```python
from build123d import *

# Parameters (mm, degrees)
DODANIE_WYCI_GNI_CIE2_DEPTH      = 3
DODANIE_WYCI_GNI_CIE2_DEPTH_BACK = 3
SZKIC2_W                         = 50
SZKIC2_H                         = 6
WYTNIJ_WYCI_GNI_CIE1_DEPTH       = 6
WYTNIJ_WYCI_GNI_CIE2_DEPTH       = 6
SZKIC4_W                         = 10
SZKIC4_H                         = 35
SZKIC4_H_2                       = 5
WYTNIJ_WYCI_GNI_CIE3_DEPTH       = 6
WYTNIJ_WYCI_GNI_CIE4_DEPTH       = 6
DODANIE_WYCI_GNI_CIE3_DEPTH      = 6
SZKIC8_R                         = 1.55
SZKIC8_R_2                       = 2.7
WYTNIJ_WYCI_GNI_CIE5_DEPTH       = 6


with BuildPart() as part:
    # Szkic1 → Dodanie-wyciągnięcie2 (new, two sides: drawn at the far end of the back side and taken through both)
    with BuildSketch(Plane(origin=(0, -418.87633849, -418.87633849), x_dir=(1, 0, 0), z_dir=(0, 1, 0)).offset(-DODANIE_WYCI_GNI_CIE2_DEPTH_BACK)):
        Polygon((-1165.368459045, -408.87633849), (-1142.368459045, -408.87633849), (-1142.368459045, -459.87633849), (-1100.368459045, -459.87633849), (-1100.368459045, -479.87633849), (-1165.368459045, -479.87633849), align=None)
    extrude(amount=DODANIE_WYCI_GNI_CIE2_DEPTH + DODANIE_WYCI_GNI_CIE2_DEPTH_BACK)

    # Szkic2 → Wytnij-wyciągnięcie1 (cut)
    with BuildSketch(Plane.XY.offset(61)):
        with Locations((-1140.368459045, -418.87633849)):
            Rectangle(SZKIC2_W, SZKIC2_H)
    extrude(amount=-WYTNIJ_WYCI_GNI_CIE1_DEPTH, mode=Mode.SUBTRACT)

    # Szkic3 → Wytnij-wyciągnięcie2 (cut)
    with BuildSketch(Plane(origin=(0, -415.87633849, 0), x_dir=(1, 0, 0), z_dir=(0, 1, 0))):
        Polygon((-1138.818459045, -55), (-1141.918459045, -55), (-1141.918459045, -51), (-1143.293459045, -51), (-1143.293459045, -49), (-1141.918459045, -49), (-1141.918459045, -48.5), (-1138.818459045, -48.5), (-1138.818459045, -49), (-1137.443459045, -49), (-1137.443459045, -51), (-1138.818459045, -51), align=None)
    extrude(amount=-WYTNIJ_WYCI_GNI_CIE2_DEPTH, mode=Mode.SUBTRACT)

    # Szkic4 → Wytnij-wyciągnięcie3 (cut)
    with BuildSketch(Plane(origin=(0, -415.87633849, 0), x_dir=(1, 0, 0), z_dir=(0, 1, 0))):
        with Locations((-1160.368459045, -17.5)):
            Rectangle(SZKIC4_W, SZKIC4_H)
        with Locations((-1160.368459045, -52.5)):
            Rectangle(SZKIC4_W, SZKIC4_H_2)
    extrude(amount=-WYTNIJ_WYCI_GNI_CIE3_DEPTH, mode=Mode.SUBTRACT)

    # Szkic5 → Wytnij-wyciągnięcie4 (cut)
    with BuildSketch(Plane(origin=(0, -415.87633849, 0), x_dir=(1, 0, 0), z_dir=(0, 1, 0))):
        Polygon((-1155.368459045, -8.168218351), (-1147.368459045, -8.168218351), (-1147.368459045, -6.793218351), (-1145.368459045, -6.793218351), (-1145.368459045, -8.168218351), (-1144.868459045, -8.168218351), (-1144.868459045, -11.268218351), (-1145.368459045, -11.268218351), (-1145.368459045, -12.643218351), (-1147.368459045, -12.643218351), (-1147.368459045, -11.268218351), (-1155.368459045, -11.268218351), align=None)
    extrude(amount=-WYTNIJ_WYCI_GNI_CIE4_DEPTH, mode=Mode.SUBTRACT)


with BuildPart() as body_2:
    # Szkic9 → Dodanie-wyciągnięcie3 (new body)
    with BuildSketch(Plane(origin=(0, -415.87633849, 0), x_dir=(1, 0, 0), z_dir=(0, 1, 0))):
        with BuildLine():
            Line((-1142.368459045, 10), (-1142.368459045, -41))
            Line((-1142.368459045, -41), (-1100.368459045, -41))
            Line((-1100.368459045, -41), (-1100.368459045, 0))
            ThreePointArc((-1100.368459045, 0), (-1103.297391233, 7.071067812), (-1110.368459045, 10))
            Line((-1110.368459045, 10), (-1142.368459045, 10))
        make_face()
    extrude(amount=-DODANIE_WYCI_GNI_CIE3_DEPTH)

    # Połącz3: union part
    add(part.part)

    # Szkic8 → Wytnij-wyciągnięcie5 (cut)
    with BuildSketch(Plane.XZ.offset(421.87633849)):
        with Locations((-1139.26479978, 35.789778966)):
            Circle(SZKIC8_R)
        with Locations((-1139.26479978, 2.789778966)):
            Circle(SZKIC8_R)
        with Locations((-1138.705640448, 20.5)):
            Circle(SZKIC8_R_2)
    extrude(amount=-WYTNIJ_WYCI_GNI_CIE5_DEPTH, mode=Mode.SUBTRACT)


solid = body_2.part
```
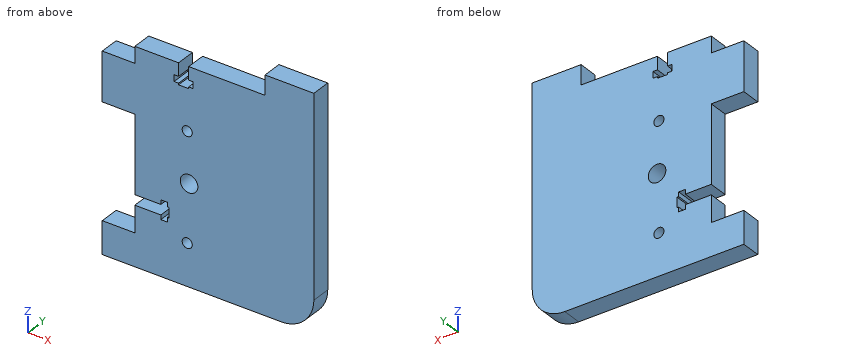
Can you work these out from the model? Positions are in its coordinate system, mm. Give positions to 0.01 mm unless a question says otherwise; leave off trailing zeros. Order: outer loops, then holes, each group sorted by start corner. A loop starts at its lowest first (then second) coordinate and runs counter-clockwise, first axis right, second up. Notation, with made-up numbers: M -34.75,-36.75 L 16.25,-36.75 A25 cw 16.25,-19.75 Z; hole C 83.5,-2 d10. An arc over 180 degrees is marked long. One line per item, written item: value.
1) For P1, Ø1.5, axis at x = -1143, y = -419, coming from the +Z side; P2, Ø4.5, axis at x = -1138.71, z = 20.5, coming from the +Y side; P3, Ø3, axis at y = -420, z = 54, coming from the -X side, each with a flat end and sliding along its axis, tell me the tip position at first contact or that it passes through.
Answer sheet:
P1: stops at z = 55
P2: passes through
P3: stops at x = -1155.37
2) I want a section at B-B, the plane z = 57. List the corners of the cut face in (x, y) for me.
Answer sheet:
outline: M -1115.37,-421.88 L -1100.37,-421.88 L -1100.37,-415.88 L -1115.37,-415.88 Z
3) Please list where these lines run through material, in increasing order: line 1 along Z through (x, y) = (-1145, -416.5); line 2 along Z through (x, y) = (-1142, -418.85); line 3 along X through (y, z) = (-416.75, 50.5).
Answer sheet:
line 1: z = -10 to 8.17, 11.27 to 55
line 2: z = -10 to 49, 51 to 55
line 3: x = -1155.37 to -1143.29, -1137.44 to -1100.37
4) I want a section at A-A, the plane z = 20.5. List the corners of the cut face in (x, y) for me.
Answer sheet:
outline: M -1155.37,-421.88 L -1141.41,-421.88 L -1141.41,-415.88 L -1155.37,-415.88 Z; M -1136.01,-421.88 L -1100.37,-421.88 L -1100.37,-415.88 L -1136.01,-415.88 Z
5) I want a section at C-C, the plane x = -1123. List the corners of the cut face in (y, z) for me, plus the area to 3 significant figures.
Answer sheet:
outline: M -421.88,-10 L -415.88,-10 L -415.88,55 L -421.88,55 Z
area: 390 mm^2
6) I want a section at D-D, the plane y = -417.75. Count the separate pieces of the cut face and the enclosed holes in it, plus the area to 3 significant figures.
Answer sheet:
separate pieces: 1
enclosed holes: 3
area: 3,790 mm^2
